```python
from build123d import *

# Parameters (mm, degrees)
F0_R     = 1
F1_DEPTH = 1.5


# Not quite as in the source:
# - ends of sketch curves that miss each other by under 0.0002 mm in the source are joined


with BuildPart() as f1:
    # F0 (on Top) → F1 (new body)
    with BuildSketch(Plane.XY):
        with BuildLine():
            Line((6.464165, -2.26795), (9.000064, -3.732051))
            ThreePointArc((9.000064, -3.732051), (9.4824259563, -3.931851665), (10.000064, -4))
            Line((10.000064, -4), (14.000064, -4))
            Line((14.000064, -4), (14.000064, 4))
            Line((14.000064, 4), (10.000064, 4))
            ThreePointArc((10.000064, 4), (9.4824257148, 3.9318516003), (9.0000636503, 3.7320506057))
            Line((9.0000636503, 3.7320506057), (6.464165, 2.267949))
            ThreePointArc((6.464165, 2.267949), (5.9817417072, 2.0681319009), (5.464038, 2.000000004))
            Line((5.464038, 2.000000004), (-5.464038, 2))
            ThreePointArc((-5.464038, 2), (-5.9817422242, 2.0681317715), (-6.4641659167, 2.2679491443))
            Line((-6.4641659167, 2.2679491443), (-9.000064, 3.73205))
            ThreePointArc((-9.000064, 3.73205), (-9.4824257148, 3.9318516003), (-10.000064, 4))
            Line((-10.000064, 4), (-14.000064, 4))
            Line((-14.000064, 4), (-14.000064, -4))
            Line((-14.000064, -4), (-10.000064, -4))
            ThreePointArc((-10.000064, -4), (-9.4824259563, -3.931851665), (-9.0000640833, -3.7320508557))
            Line((-9.0000640833, -3.7320508557), (-6.464166, -2.26795))
            ThreePointArc((-6.464166, -2.26795), (-5.9817424657, -2.0681318362), (-5.464038, -2.0000000041))
            Line((-5.464038, -2.0000000041), (5.464038, -2))
            ThreePointArc((5.464038, -2), (5.9817419487, -2.0681319656), (6.464165, -2.26795))
        make_face()
        with Locations((-12.000064, -2)):
            Circle(F0_R, mode=Mode.SUBTRACT)
        with Locations((12.000064, -2)):
            Circle(F0_R, mode=Mode.SUBTRACT)
        with Locations((-12.000064, 2)):
            Circle(F0_R, mode=Mode.SUBTRACT)
        with Locations((12.000064, 2)):
            Circle(F0_R, mode=Mode.SUBTRACT)
    extrude(amount=F1_DEPTH)


solid = f1.part
```
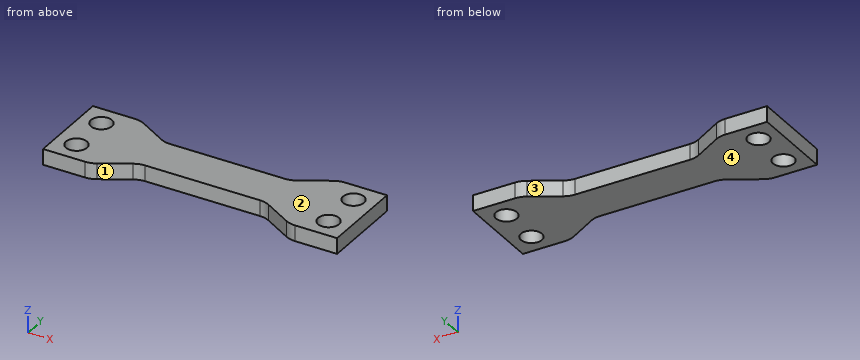
Verification items for the finished model (mm, model axes). Face numbers are marked on the shaded views. A direction names the side the tool comes from. Round coordinates to 2 decimals unless told otherwise and drop trailing zeros. Write each loop counter-clockwise with the first axis right and the second up, starting at its lowest first coordinate (ties: lowest second). Pieces come first, ordered by that corner, then holes. Notation, with made-up numbers: (45, 48.25) -> (68, 48.25) arc R17 cw to (68, 69.25) -> close; hole circle Ø11 at (73.25, 85). An arc over 180 degrees is marked (long way). Write each question's results on one line, items separated by ' | '.
Q1. Sectioned sample at A-A, the plane z = 0.7. Record the boundary of the cut face in (x, y), and give its area (3 significant figures).
Derived:
outline: (-14, -4) -> (-10, -4) arc R2 ccw to (-9, -3.73) -> (-6.46, -2.27) arc R2 cw to (-5.46, -2) -> (5.46, -2) arc R2 cw to (6.46, -2.27) -> (9, -3.73) arc R2 ccw to (10, -4) -> (14, -4) -> (14, 4) -> (10, 4) arc R2 ccw to (9, 3.73) -> (6.46, 2.27) arc R2 cw to (5.46, 2) -> (-5.46, 2) arc R2 cw to (-6.46, 2.27) -> (-9, 3.73) arc R2 ccw to (-10, 4) -> (-14, 4) -> close; hole circle Ø2 at (-12, -2); hole circle Ø2 at (-12, 2); hole circle Ø2 at (12, -2); hole circle Ø2 at (12, 2) | area: 150 mm²
Q2. Sectioned sample at D-D, the plane x = 3.75. Record the boundary of the cut face in (y, z), and give its area (3 significant figures).
Derived:
outline: (-2, 0) -> (2, 0) -> (2, 1.5) -> (-2, 1.5) -> close | area: 6.00 mm²
Q3. Sectioned sample at C-C, the plane y = -1.75. Record the boundary of the cut face in (x, z), and give its area (3 significant figures).
Derived:
outline: (-14, 0) -> (-12.97, 0) -> (-12.97, 1.5) -> (-14, 1.5) -> close; (-11.03, 0) -> (11.03, 0) -> (11.03, 1.5) -> (-11.03, 1.5) -> close; (12.97, 0) -> (14, 0) -> (14, 1.5) -> (12.97, 1.5) -> close | area: 36.2 mm²
Q4. Go/stop test with flat-tipped pins: pin 1 Ø0.8 at (x, z) = (-2, 0.5) entering from +Y; pin 2 Ø1.8 at (x, y) = (12, 2) entering from -Z. Record where each tip stops, or that it passes through.
Derived:
pin 1: stops at y = 2 | pin 2: passes through
Q5. Thickness scan on probe 1 along Y at (x, z) = (-11.5, 1.1); probe 2 along X at (y, z) = (1.75, 1); probe 3 along Y at (x, z) = (12.75, 0.8). Record the ranges inside material, lowest first.
Derived:
probe 1: y = -4 to -2.87, -1.13 to 1.13, 2.87 to 4 | probe 2: x = -14 to -12.97, -11.03 to 11.03, 12.97 to 14 | probe 3: y = -4 to -2.66, -1.34 to 1.34, 2.66 to 4
Q6. Sectioned sample at B-B, the plane x = -11.75. Record the boundary of the cut face in (y, z).
Derived:
outline: (-4, 0) -> (-2.97, 0) -> (-2.97, 1.5) -> (-4, 1.5) -> close; (-1.03, 0) -> (1.03, 0) -> (1.03, 1.5) -> (-1.03, 1.5) -> close; (2.97, 0) -> (4, 0) -> (4, 1.5) -> (2.97, 1.5) -> close
Q7. Access from +Z, -Z, +X, -X, +Y, -Y to the whole of each face (thin tool, end or side, straight path). Record for the marked faces 1 and 2.
Derived:
face 1: +Z, -Z, -Y | face 2: +Z, +X, -X, +Y, -Y
Q8. Draft check along X on the marked faces 3 and 4. Enter one of: released by +X, released by -X, zero draft, split by the parting line, or undercut.
Derived:
face 3: undercut | face 4: zero draft
